from build123d import *

# Parameters (mm, degrees)
F0_W     = 19.05
F0_H     = 12.7
F0_W_2   = 31.75
F1_DEPTH = 50.8
F3_DEPTH = 50.801
F7_DEPTH = 38.1
F8_DEPTH = 25.4


# Not quite as in the source:
# - a feature names something its author has since deleted; it is built from what else it names


with BuildPart() as f1:
    # F0 (on Top) → F1 (new body)
    with BuildSketch(Plane.XY):
        with Locations((-28.575, 6.35)):
            Rectangle(F0_W, F0_H)
        with Locations((22.225, 6.35)):
            Rectangle(F0_W_2, F0_H)
        Polygon((-19.05, 0), (0, 0), (6.35, 0), (6.35, 12.7), (-19.05, 12.7), align=None)
        Polygon((6.35, 0), (0, 0), (38.1, -38.1), (38.1, 0), align=None)
        Polygon((-38.1, -38.1), (0, 0), (-19.05, 0), (-38.1, 0), align=None)
        Polygon((38.1, -38.1), (0, 0), (-38.1, -38.1), (-19.05, -38.1), (-19.05, -25.4), (19.05, -25.4), (19.05, -38.1), align=None)
    extrude(amount=F1_DEPTH)

    # F2 (on face) → F3 (cut, through all)
    with BuildSketch(Plane(origin=(0, 12.7, 0), x_dir=(-1, 0, 0), z_dir=(0, 1, 0))):
        Polygon((-38.1, 50.8), (-38.1, 25.4), (-12.7, 50.8), align=None)
        Polygon((38.1, 50.8), (12.7, 50.8), (38.1, 25.4), align=None)
    extrude(amount=-F3_DEPTH, mode=Mode.SUBTRACT)

    # F4 (on face) → F7 (cut)
    with BuildSketch(Plane.XZ.offset(38.1)):
        Polygon((-38.1, 25.4), (-38.1, 0), (-19.05, 19.05), (-19.05, 44.45), align=None)
    extrude(amount=-F7_DEPTH, mode=Mode.SUBTRACT)

    # F5 (on face) → F8 (cut)
    with BuildSketch(Plane.XZ.offset(25.4)):
        Polygon((-19.05, 44.45), (-19.05, 19.05), (0, 38.1), (19.05, 19.05), (19.05, 44.45), (12.7, 50.8), (-12.7, 50.8), align=None)
    extrude(amount=-F8_DEPTH, mode=Mode.SUBTRACT)


solid = f1.part
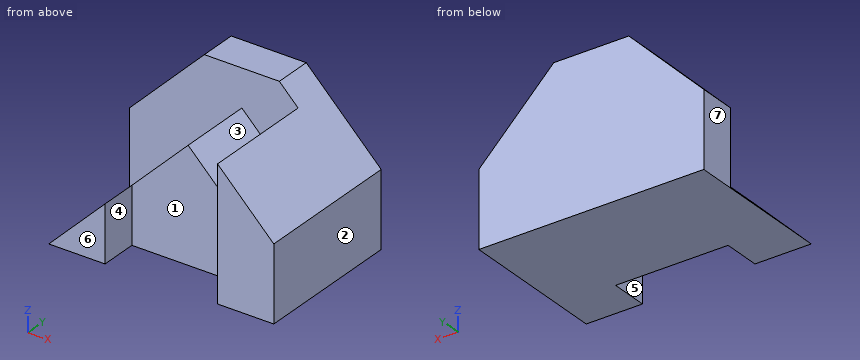
Source: CAD feature listing. Evaluate the final solid. Frame: model axes, mm. Face numbers are marked on the shaded views. A direction names the side the tool comes from. Coordinates: 2 decimals unless noted, no trailing zeros. Order: outer loops, then holes, each group sorted by start corner. A loop starts at its lowest first (then second) coordinate and runs counter-clockwise, first axis right, second up. Notation, with made-up numbers: M 38,-13 L 76,-13 A33 cw 76,19 Z; hole C 69.5,47.5 d2. An arc over 180 degrees is marked long. Write each question's results on one line, items separated by ' | '. Start each with the question number.
1. Material intervals for L1, parallel to Y at x = 3, z = 37.5; L2, parallel to Y at x = 16, z = 12.5; L3, parallel to X at y = -35, z = 15, sorted ascending.
2. Draft query along X for the marked faces 4, 5, 6 and 7. Return one class per face: +X half, -X half, draft (parallel to the pull), parting line (faces both ways), or undercut.
3. Section C-C, the plane x = 4. Return the cut outline in (y, z), then the cut area to 3 significant figures.
4. Pin query (flat end, axial travel): pin 1 (1.5 mm diameter, centred on x = -22, y = -22, fed in from -Z); pin 2 (19 mm diameter, centred on y = -25.5, z = 32, fed in from -X); pin 3 (3 mm diameter, centred on x = -24, y = 4.5, fed in from +Z); pin 4 (2 mm diameter, centred on x = -25.5, z = 23, fed in from -Y). Return the tip coordinate at first contact, or that it passes through.
5. Section A-A, the plane y = -33.5. Return the cut outline in (x, z).
6. Section D-D, the plane y = -11.5. Return the cut outline in (x, z), then the cut area to 3 significant figures.
7. Section B-B, the plane z = 13.5. Return the cut outline in (x, y), then the cut area to 3 significant figures.
8. Reachability of the marked faces 1, 2 and 3 from +Z, -Z, +X, -X, +Y, -Y: full face, straight path, thin tool, end or side. Return the list, or none.
Solution:
1) L1: 0 to 12.7 | L2: -25.4 to 12.7 | L3: -23.1 to -19.05, 19.05 to 38.1
2) face 4: undercut | face 5: undercut | face 6: draft | face 7: -X half
3) outline: M -25.4,0 L 12.7,0 L 12.7,50.8 L 0,50.8 L 0,34.1 L -25.4,34.1 Z | area: 1,510 mm²
4) pin 1: z = 0 | pin 2: x = -15.6 | pin 3: z = 41 | pin 4: y = 0
5) outline: M -38.1,0 L -19.05,0 L -19.05,19.05 Z; M 19.05,0 L 38.1,0 L 38.1,25.4 L 19.05,44.45 Z
6) outline: M -38.1,0 L 38.1,0 L 38.1,25.4 L 19.05,44.45 L 19.05,19.05 L 0,38.1 Z | area: 1,940 mm²
7) outline: M -38.1,0 L -24.6,0 L -24.6,-38.1 L -19.05,-38.1 L -19.05,-25.4 L 19.05,-25.4 L 19.05,-38.1 L 38.1,-38.1 L 38.1,12.7 L -38.1,12.7 Z | area: 2,870 mm²
8) face 1: +Z, -Z, -Y | face 2: +Z, -Z, +X, +Y, -Y | face 3: +Z, -Y
